Check sheet for the modelled part. Datum: model origin and axes. Units: mm. Coordinates: 2 decimals unless noted, no trailing zeros. Loops run counter-clockwise (first coordinate to the right, second up) from the corner with the lowest first, then second, coordinate; pieces in that order, holes last. Notation, with made-up numbers: (-21.75, 20) - (11.25, 20) arc R16 cw to (11.25, 35) - close; hole circle Ø7 at (56, -33). An arc over 180 degrees is marked (long way). Write each question's results on one line, items separated by ' | '. Start each with the question number.
1. Cross-section at B-B (y = 0.1). Record the cut outline in (x, z), and give its area (3 significant figures).
2. Thickness scan on line 1 (Z direction, x = 6, y = 0.3); line 2 (X direction, y = 0.55, z = 61); line 3 (X direction, y = -0.6, z = 72). Record the ranges inside material, lowest first. Write a range as [from, to].
3. Draft check along Z on faces 1 (the face through (-1, -0.8, 1)), 2 (the face through (92.382, -0.011, -87.871)), 3 (the face through (-49.998, -0.011, 68.418)), 4 (the face through (49.998, -0.011, 68.857)). Enter one of: released by +Z, released by -Z, zero draft, split by the parting line, or undercut.
4. Cross-section at A-A (x = -33.5). Record the cut outline in (y, z), and give its area (3 significant figures).
```python
from build123d import *

# Parameters (mm, degrees)
F1_DEPTH = 0.8


with BuildPart() as f1:
    # F0 (on Front) → F1 (new body, symmetric)
    with BuildSketch(Plane.XZ):
        with BuildLine():
            ThreePointArc((-99.9, -70), (-92.57767, -87.67767), (-74.9, -95))
            Line((-74.9, -95), (74.9, -95))
            ThreePointArc((74.9, -95), (92.57767, -87.67767), (99.9, -70))
            Line((99.9, -70), (99.9, 95))
            Line((99.9, 95), (-99.9, 95))
            Line((-99.9, 95), (-99.9, -70))
        make_face()
        with BuildLine():
            ThreePointArc((40, 78.637437), (50, 68.637437), (40, 58.637437))
            Line((40, 58.637437), (0, 58.637437))
            Line((0, 58.637437), (-40, 58.637437))
            ThreePointArc((-40, 58.637437), (-50, 68.637437), (-40, 78.637437))
            Line((-40, 78.637437), (0, 78.637437))
            Line((0, 78.637437), (40, 78.637437))
        make_face(mode=Mode.SUBTRACT)
    extrude(amount=F1_DEPTH, both=True)


solid = f1.part
```
Established:
1) outline: (-99.9, -70) arc R25 ccw to (-74.9, -95) - (74.9, -95) arc R25 ccw to (99.9, -70) - (99.9, 95) - (-99.9, 95) - close; hole (-40, 58.64) - (40, 58.64) arc R10 ccw to (40, 78.64) - (-40, 78.64) arc R10 ccw to start | area: 35,800 mm^2
2) line 1: [-95, 58.64], [78.64, 95] | line 2: [-99.9, -46.46], [46.46, 99.9] | line 3: [-99.9, -49.42], [49.42, 99.9]
3) face 1: zero draft | face 2: released by -Z | face 3: undercut | face 4: undercut
4) outline: (-0.8, -95) - (0.8, -95) - (0.8, 58.64) - (-0.8, 58.64) - close; (-0.8, 78.64) - (0.8, 78.64) - (0.8, 95) - (-0.8, 95) - close | area: 272 mm^2
